For this review, use the dimensioned drawing (mm, ordinates from the lowest corner) and the shaded views. A direction names the side the tool comes from. Round coordinates to 2 decimals unless told otherwise and drop trailing zeros. Loops run counter-clockwise (first coordinate to the right, second up) from the corner with the lowest first, then second, coordinate; pieces in that order, holes last. Notation, with made-up numbers: (17, 55.5) -> (65, 55.5) arc R29 ccw to (65, 76.5) -> close; hole circle Ø5 at (13, 68.5). An arc over 180 degrees is marked (long way). Write each question's results on one line, items separated by ' | '.
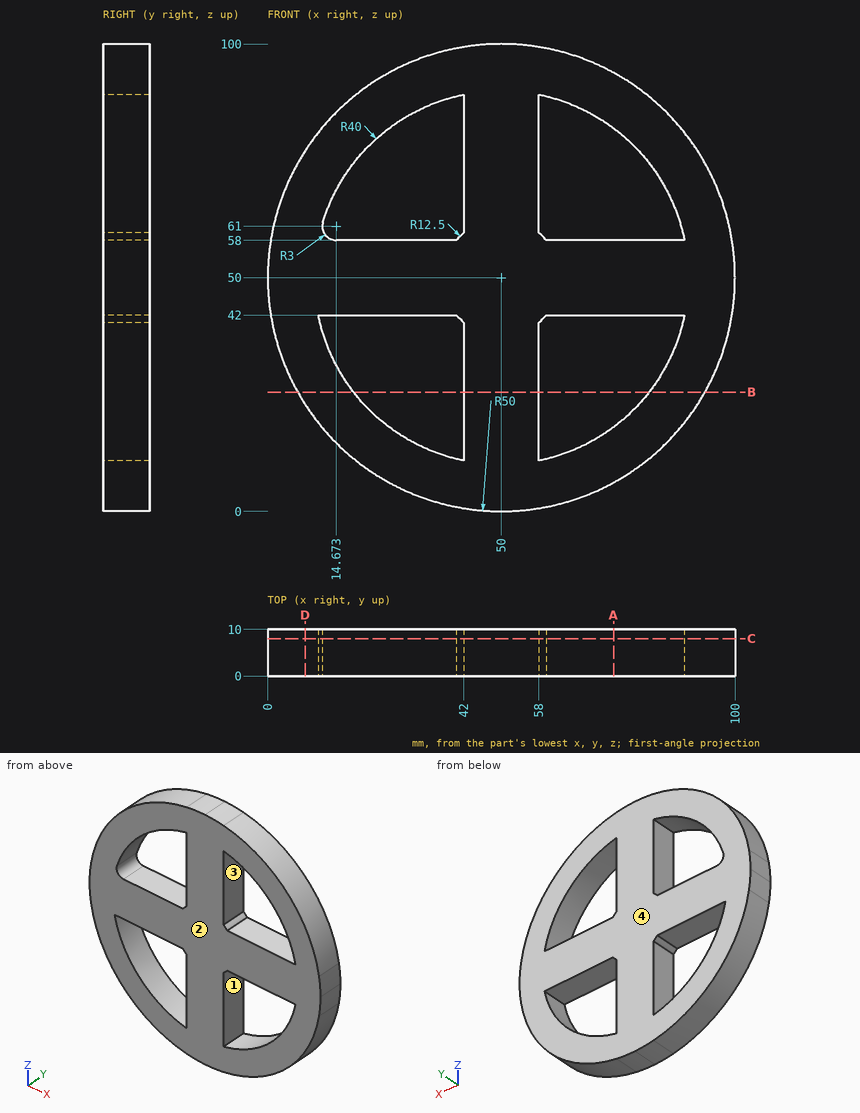
1. Consider section B-B (z = 25.5). State the section outline as (x, y) points, plus the area to 3 significant figures.
Values found:
outline: (6.41, 0) -> (18.38, 0) -> (18.38, 10) -> (6.41, 10) -> close; (42, 0) -> (58, 0) -> (58, 10) -> (42, 10) -> close; (81.62, 0) -> (93.59, 0) -> (93.59, 10) -> (81.62, 10) -> close | area: 399 mm2
2. Consider section A-A (x = 74). State the section outline as (y, z) points, plus the area to 3 significant figures.
Values found:
outline: (0, 6.14) -> (10, 6.14) -> (10, 18) -> (0, 18) -> close; (0, 42) -> (10, 42) -> (10, 58) -> (0, 58) -> close; (0, 82) -> (10, 82) -> (10, 93.86) -> (0, 93.86) -> close | area: 397 mm2
3. Consider section C-C (y = 8). State the section outline as (x, z) points.
Values found:
outline: circle Ø100 at (50, 50); hole (10.81, 42) arc R40 ccw to (42, 10.81) -> (42, 40.4) arc R12.5 cw to (40.4, 42) -> close; hole (11.81, 61.89) arc R3 ccw to (14.67, 58) -> (40.4, 58) arc R12.5 cw to (42, 59.6) -> (42, 89.19) arc R40 ccw to start; hole (58, 10.81) arc R40 ccw to (89.19, 42) -> (59.6, 42) arc R12.5 cw to (58, 40.4) -> close; hole (58, 59.6) arc R12.5 cw to (59.6, 58) -> (89.19, 58) arc R40 ccw to (58, 89.19) -> close
4. To check wall thickness, follow probe 1 along Z at (x, y) = (33, 0.5); probe 2 along X at (y, z) = (9, 21.5); probe 3 along Z at (x, y) = (81.5, 3). State the ranges of each line that lie inside material, in increasing order.
Values found:
probe 1: z = 2.98 to 13.79, 42 to 58, 86.21 to 97.02 | probe 2: x = 8.92 to 21.93, 42 to 58, 78.07 to 91.08 | probe 3: z = 11.17 to 25.35, 42 to 58, 74.65 to 88.83
5. Consider section D-D (x = 8). State the section outline as (y, z) points.
Values found:
outline: (0, 22.87) -> (10, 22.87) -> (10, 77.13) -> (0, 77.13) -> close
6. For pin 1 (5 mm diameter, centred on x = 81.5, y = 1, fed in from -Z); pin 2 (4 mm diameter, centred on x = 65.5, y = 8, fed in from -Z); pin 3 (3 mm diameter, centred on x = 28.5, y = 5, fed in from +Z), all flat-tipped, find the tip position at first contact; note any pin that passes through.
Values found:
pin 1: stops at z = 9.27 | pin 2: stops at z = 1.86 | pin 3: stops at z = 95.83
7. Draft analysis for pull direction X (two halves, no side actions). For the marked faces 1 and 2, state which applies: released by +X, released by -X, zero draft, split by the parting line, or undercut.
Values found:
face 1: undercut | face 2: zero draft
8. Tool access review of the marked faces 3 and 4: name each direction out of +Z, -Z, +X, -X, +Y, -Y from which nothing blocks a thin tool from reaching the whole face with its end or side.
Values found:
face 3: +Y, -Y | face 4: +Z, -Z, +X, -X, +Y
